Verification items for the finished model (mm, model axes). A direction names the side the tool comes from. Round coordinates to 2 decimals unless told otherwise and drop trailing zeros. Write each loop counter-clockwise with the first axis right and the second up, starting at its lowest first coordinate (ties: lowest second). Pieces come first, ordered by that corner, then holes. Notation, with made-up numbers: M 28.25,-21.75 L 41.25,-21.75 A16 cw 41.25,2.25 Z; hole C 34.25,85 d2. An arc over 180 degrees is marked long. One line per item, written item: value. Start each with the question number.
from build123d import *

# Parameters (mm, degrees)
BOSS_EXTRUDE1_DEPTH = 3
SKETCH2_W           = 3
SKETCH2_H           = 3
CUT_EXTRUDE1_DEPTH  = 3


with BuildPart() as part:
    # Sketch1 → Boss-Extrude1 (new body)
    with BuildSketch(Plane(origin=(0, 0, 0), x_dir=(1, 0, 0), z_dir=(0, 1, 0))):
        Polygon((-5.5, 0), (13.5, 10.5), (13.5, 12.5), (-10.5, 12.5), (-10.5, 8), (-13.5, 8), (-13.5, 2), (-10.5, 2), (-10.5, -2), (-13.5, -2), (-13.5, -8), (-10.5, -8), (-10.5, -12.5), (13.5, -12.5), (13.5, -10.5), align=None)
    extrude(amount=BOSS_EXTRUDE1_DEPTH)

    # Sketch2 → Cut-Extrude1 (cut)
    with BuildSketch(Plane(origin=(0, 3, 0), x_dir=(1, 0, 0), z_dir=(0, 1, 0))):
        with Locations((-6, 5)):
            Rectangle(SKETCH2_W, SKETCH2_H)
        with Locations((-6, -5)):
            Rectangle(SKETCH2_W, SKETCH2_H)
    extrude(amount=-CUT_EXTRUDE1_DEPTH, mode=Mode.SUBTRACT)


solid = part.part
1) Cross-section at B-B (z = -6). Record the boundary of the cut face in (x, y), then the cut area to 3 significant figures.
2) Thickness scan on line 1 (Z direction, x = -7.25, y = 1.5); line 2 (X direction, y = 1.1, z = 6); line 3 (Z direction, x = 3.25, y = 2.35). Record the ranges inside material, lowest first.
3) Cross-section at A-A (y = 2.3). Record the boundary of the cut face in (x, z), then the cut area to 4 significant figures.
4) Mould release check, pull along X, two halves, no side actions. Record for faces 1 (the flat face through (-10.5, 1, 10)), 2 (the flat face through (-12, 1, -2)), 3 (the flat face through (-7.5, 2, 5)): pulls with the +X half, pulls with the -X half, needs draft (parallel to the pull), parting line crosses it, or undercut.
5) Gauge pin test, flat ends, axial feed: pin 1 Ø1 at (y, z) = (0.5, 1) entering from -X; pin 2 Ø6 at (x, z) = (6, -2) entering from -Y. Record the tip position at first contact, or that the pin passes through.
6) Cross-section at C-C (x = 9.75). Record the boundary of the cut face in (y, z), then the cut area to 3 significant figures.
7) Cross-section at D-D (z = -9.25). Record the boundary of the cut face in (x, y).
8) Access from +Z, -Z, +X, -X, +Y, -Y to the whole of each face (thin tool, end or side, straight path). Record for faces 4 (the flat face through (-10.5, 1, 0)), 5 (the flat face through (-6, 2, 6.5)), 6 (the flat face through (-10.5, 1, -10)).
Results below:
1. outline: M -13.5,0 L -7.5,0 L -7.5,3 L -13.5,3 Z; M -4.5,0 L 5.36,0 L 5.36,3 L -4.5,3 Z
1. area: 47.6 mm²
2. line 1: z = -12.5 to -6.5, -3.5 to 3.5, 6.5 to 12.5
2. line 2: x = -13.5 to -7.5, -4.5 to 5.36
2. line 3: z = -12.5 to -4.84, 4.84 to 12.5
3. outline: M -13.5,-8 L -10.5,-8 L -10.5,-12.5 L 13.5,-12.5 L 13.5,-10.5 L -5.5,0 L 13.5,10.5 L 13.5,12.5 L -10.5,12.5 L -10.5,8 L -13.5,8 L -13.5,2 L -10.5,2 L -10.5,-2 L -13.5,-2 Z; hole M -7.5,-6.5 L -4.5,-6.5 L -4.5,-3.5 L -7.5,-3.5 Z; hole M -7.5,3.5 L -4.5,3.5 L -4.5,6.5 L -7.5,6.5 Z
3. area: 418.5 mm²
4. face 1: pulls with the -X half
4. face 2: needs draft
4. face 3: undercut
5. pin 1: stops at x = -10.5
5. pin 2: passes through
6. outline: M 0,-12.5 L 3,-12.5 L 3,-8.43 L 0,-8.43 Z; M 0,8.43 L 3,8.43 L 3,12.5 L 0,12.5 Z
6. area: 24.4 mm²
7. outline: M -10.5,0 L 11.24,0 L 11.24,3 L -10.5,3 Z
8. face 4: -X, +Y, -Y
8. face 5: +Y, -Y
8. face 6: -Z, -X, +Y, -Y
